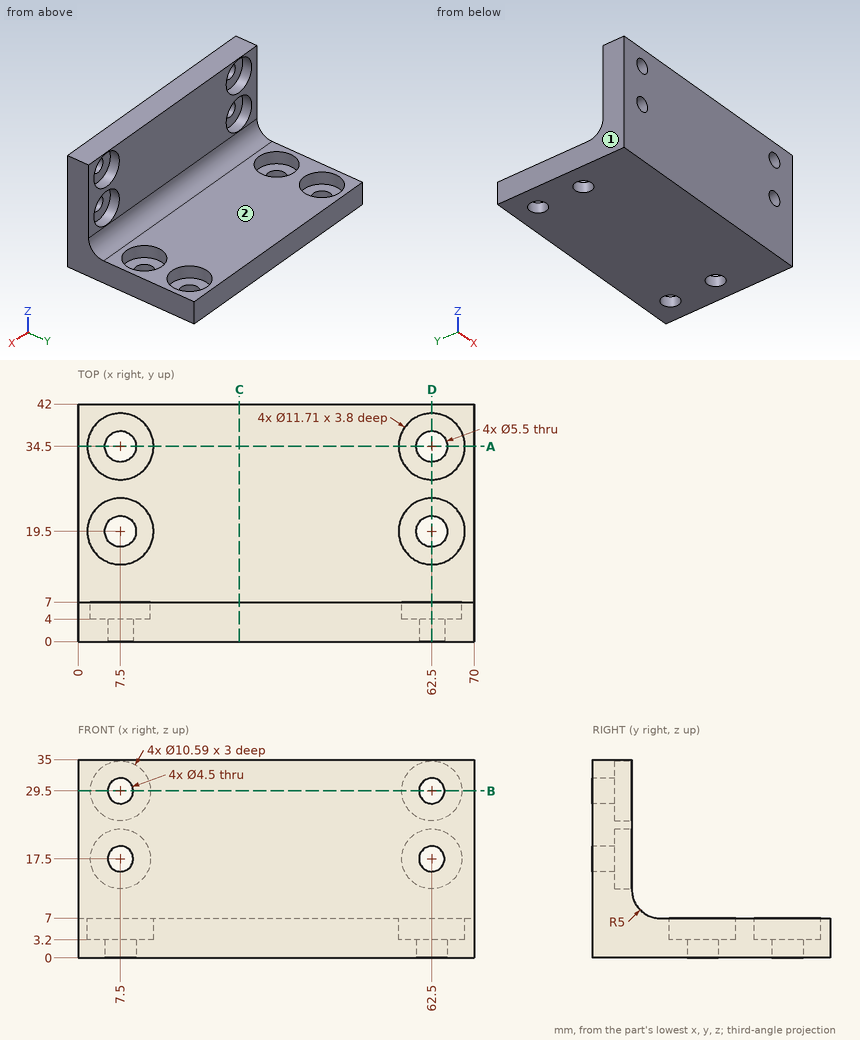
Design review of the part shown in the three views and the two pictorial views. Dimensions are in mm from the part's minimum x, y and z. A direction names the side the tool comes from. Round coordinates to 2 decimals unless told otherwise and drop trailing zeros. Loops run counter-clockwise (first coordinate to the right, second up) from the corner with the lowest first, then second, coordinate; pieces in that order, holes last. Notation, with made-up numbers: (56, -13) -> (109, -13) arc R17 ccw to (109, 3) -> close; hole circle Ø5 at (63.25, 70.25). An arc over 180 degrees is marked (long way). Answer as a JSON object with one key per item and string values. Group by question number.
1) We need section B-B on z = 29.5. Write out the cut boundary in (x, y) (3 decimals).
2) We need section C-C on x = 28.5. Write out the cut boundary in (y, z).
3) For the marked faces 1 and 2, list the 3-axis set-ups (+Z, -Z, +X, -X, +Y, -Y) from which the entire face can be reached by the end or side of a thin tool; tool diameter is ignored.
4) For pin 1 Ø4.5 at (x, y) = (62.5, 19.5) entering from -Z; pin 2 Ø15 at (x, y) = (62.5, 34.5) entering from +Z; pin 3 Ø10.5 at (x, y) = (62.5, 19.5) entering from +Z; pin 4 Ø3 at (x, z) = (8.5, 19.5) entering from +Y, all flat-tipped, find the tip position at first contact; note any pin that passes through.
5) For line 1 (Y direction, x = 7.5, z = 1.4); line 2 (Z direction, x = 62.5, y = 5.5) (3 decimals); line 3 (Z direction, x = 7.5, y = 1.4), list the stretches that pass through material, from the lowest coordinate up. Write a range as [from, to].
6) We need section A-A on y = 34.5. Write out the cut boundary in (x, z) (3 decimals).
7) We need section D-D on x = 62.5. Give the number of separate pieces and of enclosed holes in the cut face, then the cut area to 3 significant figures.
Result set:
{
 "1": {"outline": "(0, 0) -> (5.25, 0) -> (5.25, 4) -> (2.205, 4) -> (2.205, 7) -> (0, 7) -> close; (9.75, 0) -> (60.25, 0) -> (60.25, 4) -> (57.205, 4) -> (57.205, 7) -> (12.795, 7) -> (12.795, 4) -> (9.75, 4) -> close; (64.75, 0) -> (70, 0) -> (70, 7) -> (67.795, 7) -> (67.795, 4) -> (64.75, 4) -> close"},
 "2": {"outline": "(0, 0) -> (42, 0) -> (42, 7) -> (12, 7) arc R5 cw to (7, 12) -> (7, 35) -> (0, 35) -> close"},
 "3": {"face 1": "+Z, -Z, -X, +Y, -Y", "face 2": "+Z, +X, -X, +Y"},
 "4": {"pin 1": "through", "pin 2": "z = 7", "pin 3": "z = 3.2", "pin 4": "y = 4"},
 "5": {"line 1": "[0, 16.75], [22.25, 31.75], [37.25, 42]", "line 2": "[0, 12.205], [22.795, 24.205], [34.795, 35]", "line 3": "[0, 15.25], [19.75, 27.25], [31.75, 35]"},
 "6": {"outline": "(0, 0) -> (4.75, 0) -> (4.75, 3.2) -> (1.645, 3.2) -> (1.645, 7) -> (0, 7) -> close; (10.25, 0) -> (59.75, 0) -> (59.75, 3.2) -> (56.645, 3.2) -> (56.645, 7) -> (13.355, 7) -> (13.355, 3.2) -> (10.25, 3.2) -> close; (65.25, 0) -> (70, 0) -> (70, 7) -> (68.355, 7) -> (68.355, 3.2) -> (65.25, 3.2) -> close"},
 "7": {"separate pieces": "5", "enclosed holes": "0", "area": "272 mm²"}
}
